The listing builds one solid part. Answer for the finished solid, in the listing's coordinates (mm). A direction names the side the tool comes from. Round coordinates to 2 decimals unless told otherwise and drop trailing zeros. Order: outer loops, then holes, each group sorted by start corner. A loop starts at its lowest first (then second) coordinate and runs counter-clockwise, first axis right, second up. Notation, with made-up numbers: (88.5, 5) - (122.5, 5) arc R15 ccw to (122.5, 27) - close; hole circle Ø10 at (-0.75, -38). An arc over 180 degrees is marked (long way). Use CSV: the item, a comma, the result in double quotes. Start each with the question number.
Item 1: Find section A-A, the plane x = 0. Give the vertices of the cut face in (y, z).
Item 2: Flat-ended cylindrical pins translate along their axes: P1, Ø1, axis at y = 3.5, z = 1, coming from the -X side; P2, Ø4, axis at x = 11.89, z = -3.86, coming from the +Y side; P3, Ø8, axis at y = 14, z = -4, coming from the +X side. Find the tip coordinate at first contact, or state that the pin passes through.
Item 3: Find section D-D, the plane y = 14.25. Give the vertices of the cut face in (x, z).
Item 4: Determine the mould class of faces 4 (the cylindrical face through (-6.979, 8.522, 11.772)), 5 (the flat face through (4, 17, -4)), 6 (the cylindrical face through (18.548, 8.112, 4.119)) for opening direction Z: +Z half, -Z half, draft (parallel to the pull), parting line (faces both ways), or undercut.
Item 5: For faces 1 (the cylindrical face through (3.905, 14.218, 0.867)), 2 (the cylindrical face through (13.587, 8.522, -3.937)), 3 (the flat face through (0, 7, 0)), determine the directions among +Z, -Z, +X, -X, +Y, -Y from which every point of the face is accessible in a straight line to the end or side of a thin tool.
Item 6: Straight lines are drawn through the part: line 1 along X through (y, z) = (2.85, 0); line 2 along Z through (x, y) = (-6, 3.5); line 3 along X through (y, z) = (16, 10.5). For each, find the intervals that lie inside material, in ascending order. Write a range as [from, to].
Item 7: Find section B-B, the plane y = 6.25. Give the vertices of the cut face in (x, z).
Item 8: Find section C-C, the plane z = -5. Count the separate pieces of the cut face and the enclosed holes in it, plus the area to 3 significant figures.
```python
from build123d import *

# Parameters (mm, degrees)
CSK_FOR_M3_HEX_SOCKET_COUNTERSUNK_HEAD_S_D           = 3.4
CSK_FOR_M3_HEX_SOCKET_COUNTERSUNK_HEAD_S_CSINK_D     = 6.94
CSK_FOR_M3_HEX_SOCKET_COUNTERSUNK_HEAD_S_CSINK_ANGLE = 90
SKETCH6_R                                            = 7.5
CUT_EXTRUDE1_DEPTH                                   = 5
CHAMFER1_SIZE                                        = 3
CHAMFER2_SIZE                                        = 1
CHAMFER3_SIZE                                        = 0.5


with BuildPart() as part:
    # Sketch1 → Revolve1 (revolve)
    with BuildSketch(Plane.XY, mode=Mode.PRIVATE) as revolve1_sk:
        Polygon((17, 0), (19, 0), (19, 17), (4, 17), (4, 12), (0, 12), (0, 2), (17, 2), align=None)
    revolve(revolve1_sk.sketch.rotate(Axis((0, 0, 0), (0, 1, 0)), 90), axis=Axis((0, 0, 0), (0, 1, 0)))

    # CSK for M3 Hex Socket Countersunk Head Screw1 (through all)
    with Locations(Plane(origin=(0, 17, 0), x_dir=(1, 0, 0), z_dir=(0, 1, 0))):
        with Locations((-11.888206454, 3.86271243), (0, 12.5), (11.888206454, 3.86271243), (7.347315654, -10.11271243), (-7.347315654, -10.11271243)):
            CounterSinkHole(CSK_FOR_M3_HEX_SOCKET_COUNTERSUNK_HEAD_S_D / 2, CSK_FOR_M3_HEX_SOCKET_COUNTERSUNK_HEAD_S_CSINK_D / 2, counter_sink_angle=CSK_FOR_M3_HEX_SOCKET_COUNTERSUNK_HEAD_S_CSINK_ANGLE)

    # Sketch6 → Cut-Extrude1 (cut)
    with BuildSketch(Plane.XZ.offset(-2)):
        with Locations(Location((0, 0, 0), (0, 0, 270))):
            Circle(SKETCH6_R)
    extrude(amount=-CUT_EXTRUDE1_DEPTH, mode=Mode.SUBTRACT)

    # Chamfer1
    chamfer1_edges = [part.edges().sort_by_distance(p)[0] for p in [
        (0, 7, 7.5),
    ]]
    chamfer(chamfer1_edges, length=CHAMFER1_SIZE)

    # Chamfer2
    chamfer2_edges = [part.edges().sort_by_distance(p)[0] for p in [
        (0, 17, 19),
    ]]
    chamfer(chamfer2_edges, length=CHAMFER2_SIZE)

    # Chamfer3
    chamfer3_edges = [part.edges().sort_by_distance(p)[0] for p in [
        (0, 17, 4),
    ]]
    chamfer(chamfer3_edges, length=CHAMFER3_SIZE)


solid = part.part
```
Worked out:
1,outline,"(0, -19) - (16, -19) - (17, -18) - (17, -15.97) - (15.23, -14.2) - (2, -14.2) - (2, -17) - (0, -17) - close; (0, 17) - (2, 17) - (2, 7.5) - (4, 7.5) - (7, 4.5) - (7, -4.5) - (4, -7.5) - (2, -7.5) - (2, -10.8) - (15.23, -10.8) - (17, -9.03) - (17, -4.5) - (16.5, -4) - (12, -4) - (12, 4) - (16.5, 4) - (17, 4.5) - (17, 18) - (16, 19) - (0, 19) - close"
2,P1,"stops at x = -18.99"
2,P2,"stops at y = 15.53"
2,P3,"stops at x = 19"
3,outline,"circle Ø38 at (0, 0); hole circle Ø3.4 at (-11.89, -3.86); hole circle Ø3.4 at (-7.35, 10.11); hole circle Ø8 at (0, 0); hole circle Ø3.4 at (0, -12.5); hole circle Ø3.4 at (7.35, 10.11); hole circle Ø3.4 at (11.89, -3.86)"
4,face 4,"undercut"
4,face 5,"draft"
4,face 6,"parting line"
5,face 1,"+Y"
5,face 2,"+Y, -Y"
5,face 3,"-Y"
6,line 1,"x = [-19, -7.5], [7.5, 19]"
6,line 2,"z = [-18.03, -4.5], [4.5, 9.08], [11.15, 18.03]"
6,line 3,"x = [-15.84, -9.79], [-4.91, 4.91], [9.79, 15.84]"
7,outline,"circle Ø38 at (0, 0); hole circle Ø3.4 at (-11.89, -3.86); hole circle Ø3.4 at (-7.35, 10.11); hole circle Ø10.5 at (0, 0); hole circle Ø3.4 at (0, -12.5); hole circle Ø3.4 at (7.35, 10.11); hole circle Ø3.4 at (11.89, -3.86)"
8,separate pieces,"3"
8,enclosed holes,"0"
8,area,"434 mm²"
